from build123d import *

# Parameters (mm, degrees)
F1_DEPTH      = 10.16
F2_R          = 7.62
F3_DEPTH      = 6.35
F3_DEPTH_BACK = 19.05
F4_R          = 6.35
F5_DEPTH      = 25.401


with BuildPart() as f1:
    # F0 (on Right) → F1 (new body)
    with BuildSketch(Plane.YZ):
        Polygon((1.410603, 9.427101), (-7.458808, 5.935168), (-8.86941, -3.491933), (-1.410603, -9.427101), (7.458808, -5.935168), (8.86941, 3.491933), align=None)
    extrude(amount=F1_DEPTH)

    # F2 (on face) → F3 (join, two sides)
    with BuildSketch(Plane.YZ.offset(10.16)) as f3_sk:
        Circle(F2_R)
    extrude(amount=F3_DEPTH)
    extrude(f3_sk.sketch, amount=-F3_DEPTH_BACK)

    # F4 (on face) → F5 (cut, through all)
    with BuildSketch(Plane(origin=(-8.89, 0, 0), x_dir=(0, -1, 0), z_dir=(-1, 0, 0))):
        Circle(F4_R)
    extrude(amount=-F5_DEPTH, mode=Mode.SUBTRACT)


solid = f1.part
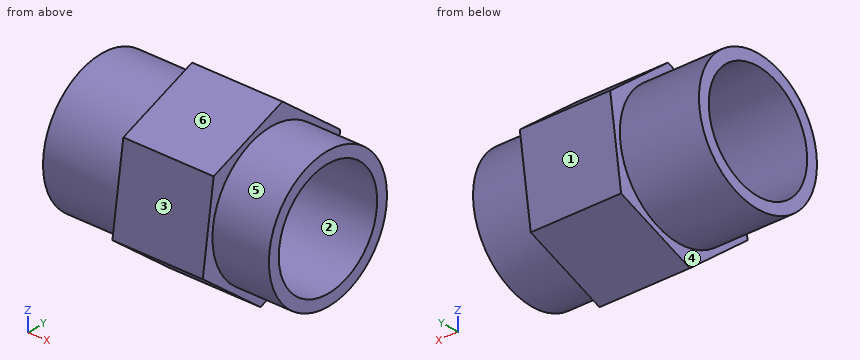
Input: part model. Units: mm. Frame: model coordinates. Face numbers are marked on the shaded views. A direction names the side the tool comes from. Give positions to 0.01 mm unless a question says otherwise; leave off trailing zeros. Write each loop counter-clockwise with the first axis right and the second up, starting at its lowest first coordinate (ties: lowest second). Pieces come first, ordered by that corner, then holes.
Q1. First-contact query: P1, Ø5, axis at x = 9, z = -5, coming from the +Y side; P2, Ø5, axis at x = 2.5, y = -3, coming from the -Z side; P3, Ø1.5, axis at x = 3.5, z = -6, coming from the +Y side. Flat tips, straight axial feed; report the tip coordinate or a pass-through.
Q2. Pull-direction query (Y, two-part tool) for the marked faces 1, 2 and 3; classes: pulls with the +Y half, pulls with the -Y half, needs draft (parallel to the pull), parting line crosses it, or undercut.
Q3. Material intervals for probe 1 along Z at (x, y) = (7.75, 0); probe 2 along Z at (x, y) = (-5.75, 1.75); probe 3 along Y at (x, z) = (-0.75, -0.5), sorted ascending.
Q4. Set-up query: the marked faces 4, 5 and 6. Return all of +Z, -Z, +X, -X, +Y, -Y with unobstructed straight access to the full face (end or side cutting, diameter ignored); none if empty.
Q5. Section C-C, the plane z = 2.75. Output: boundary loops of the cut face in (x, y), plus the area to 3 significant figures.
Q6. Section D-D, the plane x = -0.5. Output: boundary loops of the cut face in (y, z), plus the area to 3 significant figures.
Q7. Section A-A, the plane x = 6.5. Output: boundary loops of the cut face in (y, z), plus the area to 3 significant figures.
Q8. Section B-B, the plane y = 0. Output: boundary loops of the cut face in (x, z).
Filled in:
1. P1: stops at y = 7.97
1. P2: stops at z = -9.43
1. P3: stops at y = 7.56
2. face 1: pulls with the +Y half
2. face 2: undercut
2. face 3: pulls with the -Y half
3. probe 1: z = -8.87 to -6.35, 6.35 to 8.87
3. probe 2: z = -7.42 to -6.1, 6.1 to 7.42
3. probe 3: y = -7.6 to -6.33, 6.33 to 7.6
4. face 4: -X
4. face 5: +X
4. face 6: +Z, +X, -X, -Y
5. outline: (-8.89, -7.11) - (0, -7.11) - (0, -7.94) - (10.16, -7.94) - (10.16, -7.11) - (16.51, -7.11) - (16.51, -5.72) - (-8.89, -5.72) - close; (-8.89, 5.72) - (16.51, 5.72) - (16.51, 7.11) - (10.16, 7.11) - (10.16, 8.76) - (0, 8.76) - (0, 7.11) - (-8.89, 7.11) - close
5. area: 95.5 mm2
6. outline: circle Ø15.24 at (0, 0); hole circle Ø12.7 at (0, 0)
6. area: 55.7 mm2
7. outline: (-8.87, -3.49) - (-1.41, -9.43) - (7.46, -5.94) - (8.87, 3.49) - (1.41, 9.43) - (-7.46, 5.94) - close; hole circle Ø12.7 at (0, 0)
7. area: 109 mm2
8. outline: (-8.89, -7.62) - (0, -7.62) - (0, -8.87) - (10.16, -8.87) - (10.16, -7.62) - (16.51, -7.62) - (16.51, -6.35) - (-8.89, -6.35) - close; (-8.89, 6.35) - (16.51, 6.35) - (16.51, 7.62) - (10.16, 7.62) - (10.16, 8.87) - (0, 8.87) - (0, 7.62) - (-8.89, 7.62) - close
